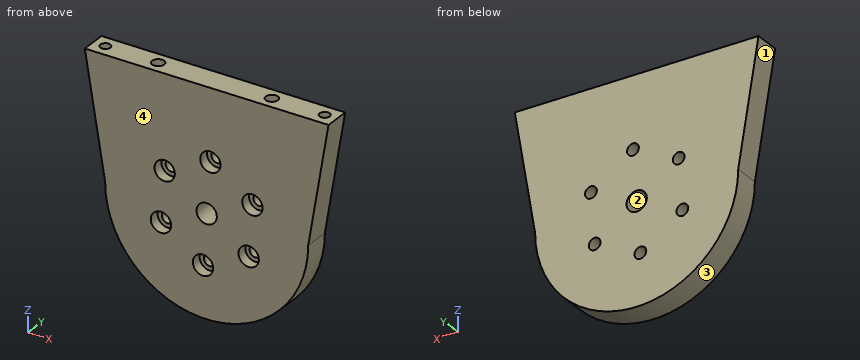
from build123d import *

# Parameters (mm, degrees)
PLACA_J5_START           = -3.175
PLACA_J5_DEPTH           = 6.35
PLACA_J5_REDONDEO_START  = -3.175
CROQUIS9_R               = 25
PLACA_J5_REDONDEO_DEPTH  = 6.35
BARRENOS_SALIDA_M5_START = -3.175
CROQUIS10_R              = 1.45
CROQUIS10_R_2            = 2.5
BARRENOS_SALIDA_M5_DEPTH = 6.35
REFRENTADO_M2_5_START    = -3.175
CROQUIS11_R              = 2.5
REFRENTADO_M2_5_DEPTH    = 2.6
ROSCA_M3_CANTO_START     = 357.55
CROQUIS12_R              = 1.25
ROSCA_M3_CANTO_DEPTH     = 9
PASADORES_D3_START       = 359.55
CROQUIS13_R              = 1.5
PASADORES_D3_DEPTH       = 7


with BuildPart() as part:
    # Croquis8 → Placa_J5 (new body)
    with BuildSketch(Plane(origin=(0, 0, 0), x_dir=(1, 0, 0), z_dir=(0, 1, 0)).offset(PLACA_J5_START)):
        Polygon((127.4, -336.55), (177.4, -336.55), (182.4, -366.55), (122.4, -366.55), align=None)
    extrude(amount=PLACA_J5_DEPTH)

    # Croquis9 → Placa_J5_redondeo (add)
    with BuildSketch(Plane(origin=(0, 0, 0), x_dir=(1, 0, 0), z_dir=(0, 1, 0)).offset(PLACA_J5_REDONDEO_START)):
        with Locations((152.4, -336.55)):
            Circle(CROQUIS9_R)
    extrude(amount=PLACA_J5_REDONDEO_DEPTH)

    # Croquis10 → Barrenos_salida_M5 (cut)
    with BuildSketch(Plane(origin=(0, 0, 0), x_dir=(1, 0, 0), z_dir=(0, 1, 0)).offset(BARRENOS_SALIDA_M5_START)):
        with Locations(Location((163.653984643, -341.990388742, 0), (0, 0, 270))):
            Circle(CROQUIS10_R)
        with Locations(Location((153.315477464, -349.016430965, 0), (0, 0, 270))):
            Circle(CROQUIS10_R)
        with Locations(Location((142.061492822, -343.576042223, 0), (0, 0, 270))):
            Circle(CROQUIS10_R)
        with Locations(Location((141.146015357, -331.109611258, 0), (0, 0, 270))):
            Circle(CROQUIS10_R)
        with Locations(Location((151.484522536, -324.083569035, 0), (0, 0, 270))):
            Circle(CROQUIS10_R)
        with Locations(Location((162.738507178, -329.523957777, 0), (0, 0, 270))):
            Circle(CROQUIS10_R)
        with Locations(Location((152.4, -336.55, 0), (0, 0, 270))):
            Circle(CROQUIS10_R_2)
    extrude(amount=BARRENOS_SALIDA_M5_DEPTH, mode=Mode.SUBTRACT)

    # Croquis11 → Refrentado_M2-5 (cut)
    with BuildSketch(Plane(origin=(0, 0, 0), x_dir=(1, 0, 0), z_dir=(0, 1, 0)).offset(REFRENTADO_M2_5_START)):
        with Locations(Location((163.653984643, -341.990388742, 0), (0, 0, 270))):
            Circle(CROQUIS11_R)
        with Locations(Location((153.315477464, -349.016430965, 0), (0, 0, 270))):
            Circle(CROQUIS11_R)
        with Locations(Location((142.061492822, -343.576042223, 0), (0, 0, 270))):
            Circle(CROQUIS11_R)
        with Locations(Location((141.146015357, -331.109611258, 0), (0, 0, 270))):
            Circle(CROQUIS11_R)
        with Locations(Location((151.484522536, -324.083569035, 0), (0, 0, 270))):
            Circle(CROQUIS11_R)
        with Locations(Location((162.738507178, -329.523957777, 0), (0, 0, 270))):
            Circle(CROQUIS11_R)
    extrude(amount=REFRENTADO_M2_5_DEPTH, mode=Mode.SUBTRACT)

    # Croquis12 → Rosca_M3_canto (cut)
    with BuildSketch(Plane.XY.offset(ROSCA_M3_CANTO_START)):
        with Locations((125.4, 0)):
            Circle(CROQUIS12_R)
        with Locations((179.4, 0)):
            Circle(CROQUIS12_R)
    extrude(amount=ROSCA_M3_CANTO_DEPTH, mode=Mode.SUBTRACT)

    # Croquis13 → Pasadores_D3 (cut)
    with BuildSketch(Plane.XY.offset(PASADORES_D3_START)):
        with Locations((138.4, 0)):
            Circle(CROQUIS13_R)
        with Locations((166.4, 0)):
            Circle(CROQUIS13_R)
    extrude(amount=PASADORES_D3_DEPTH, mode=Mode.SUBTRACT)


solid = part.part
CAD build for the part. Positions are in the model's coordinates, mm. Face numbers are marked on the shaded views. Round coordinates to 2 decimals unless told otherwise and drop trailing zeros. Loops run counter-clockwise (first coordinate to the right, second up) from the corner with the lowest first, then second, coordinate; pieces in that order, holes last. Notation, with made-up numbers: M 61.5,-15.5 L 76.5,-15.5 A23 ccw 76.5,-1.5 Z; hole C -24,12 d2. An arc over 180 degrees is marked long. One line per question, with ' | ' between items. Start each with the question number.
Item 1: Wall check: line 1 (Z direction, x = 153, y = -1.5); line 2 (X direction, y = -0.75, z = 362); line 3 (Y direction, x = 125.4, z = 362.5) (3 decimals). Give the ranges that are in metal, low to high.
Item 2: Pin check, flat tips, straight feed: pin 1 Ø3 at (x, y) = (179, -0.5) entering from +Z; pin 2 Ø2 at (y, z) = (0.5, 330) entering from +X; pin 3 Ø2.5 at (x, y) = (138.4, 0) entering from -Z; pin 4 Ø1.5 at (x, z) = (164.5, 341) entering from -Y (3 decimals). Stop position of each tip, or through.
Item 3: Cut at B-B, the plane x = 179.4. Write the cut outline in (y, z) (3 decimals), plus the area to 3 significant figures.
Item 4: Cut at A-A, the plane y = -2.5. Write the cut outline in (x, z).
Item 5: Cut at C-C, the plane z = 317.5. Write the cut outline in (x, y) (3 decimals).
Item 6: Two-plate mould, pull along X, no slides. Class the marked faces 1, 2, 3 and 4: pulls with the +X half, pulls with the -X half, needs draft (parallel to the pull), parting line crosses it, or undercut.
Responses:
1) line 1: z = 311.56 to 322.1, 326.07 to 334.12, 338.98 to 346.54, 351.5 to 366.55 | line 2: x = 123.16 to 124.4, 126.4 to 137.1, 139.7 to 165.1, 167.7 to 178.4, 180.4 to 181.64 | line 3: y = -3.175 to -1.25, 1.25 to 3.175
2) pin 1: stops at z = 366.55 | pin 2: stops at x = 176.78 | pin 3: stops at z = 315.05 | pin 4: stops at y = -0.575
3) outline: M -3.175,348.55 L 3.175,348.55 L 3.175,366.55 L 1.25,366.55 L 1.25,357.55 L -1.25,357.55 L -1.25,366.55 L -3.175,366.55 Z | area: 91.8 mm²
4) outline: M 122.4,366.55 L 127.4,336.55 A25 ccw 177.4,336.55 L 182.4,366.55 Z; hole C 141.15,331.11 d5; hole C 142.06,343.58 d5; hole C 151.48,324.08 d5; hole C 152.4,336.55 d5; hole C 153.32,349.02 d5; hole C 162.74,329.52 d5; hole C 163.65,341.99 d5
5) outline: M 136.211,-3.175 L 168.589,-3.175 L 168.589,3.175 L 136.211,3.175 Z
6) face 1: pulls with the -X half | face 2: undercut | face 3: parting line crosses it | face 4: needs draft
